CAD build for the part. Positions are in the model's coordinates, mm. Coordinates: 2 decimals unless noted, no trailing zeros. Write each loop counter-clockwise with the first axis right and the second up, starting at its lowest first coordinate (ties: lowest second). Pieces come first, ordered by that corner, then holes. Notation, with made-up numbers: (81, -8) -> (132, -8) arc R24 cw to (132, 23) -> close; hole circle Ø8 at (-28, 69). An arc over 180 degrees is marked (long way). Answer as CSV lines item,"result".
Autodesk Inventor part; units mm, degrees
ref_plane "YZ Plane" through (0, 0, 0) normal (1, 0, 0) x (0, 1, 0)
ref_plane "XZ Plane" through (0, 0, 0) normal (0, 1, 0) x (-1, 0, 0)
ref_plane "XY Plane" through (0, 0, 0) normal (0, 0, 1) x (1, 0, 0)
sketch "Sketch1" plane through (0, 0, 0) normal (1, 0, 0) x (0, 1, 0)
  line L0 (21.2, 0) -> (21.2, -3)
  line L1 (42.4, 0) -> (42.4, -3)
  line L2 (63.6, 0) -> (63.6, -3)
  line L3 (84.8, 0) -> (84.8, -3)
  line L4 (-3, -21.2) -> (3, -21.2)
  line L5 (-3, -42.4) -> (3, -42.4)
  line L6 (-3, -63.6) -> (3, -63.6)
  line L7 (-3, -84.8) -> (3, -84.8)
  line L8 (21.2, -106) -> (21.2, -103)
  line L9 (42.4, -106) -> (42.4, -103)
  line L10 (63.6, -106) -> (63.6, -103)
  line L11 (84.8, -106) -> (84.8, -103)
  line L12 (109, -84.8) -> (103, -84.8)
  line L13 (109, -63.6) -> (103, -63.6)
  line L14 (109, -42.4) -> (103, -42.4)
  line L15 (109, -21.2) -> (103, -21.2)
  line L16 (3, -103) -> (3, -84.8)
  line L17 (3, -63.6) -> (3, -42.4)
  line L18 (3, -21.2) -> (3, -3)
  line L19 (103, -3) -> (103, -21.2)
  line L20 (103, -42.4) -> (103, -63.6)
  line L21 (103, -84.8) -> (103, -103)
  line L22 (21.2, -103) -> (3, -103)
  line L23 (84.8, -106) -> (63.6, -106)
  line L24 (42.4, -106) -> (21.2, -106)
  line L25 (103, -103) -> (84.8, -103)
  line L26 (63.6, -103) -> (42.4, -103)
  line L27 (103, -3) -> (103, 0)
  line L28 (3, -3) -> (3, 0)
  line L29 (3, 0) -> (21.2, 0)
  line L30 (21.2, -3) -> (42.4, -3)
  line L31 (63.6, -3) -> (84.8, -3)
  line L32 (42.4, 0) -> (63.6, 0)
  line L33 (84.8, 0) -> (103, 0)
  line L34 (-3, -21.2) -> (-3, -42.4)
  line L35 (-3, -63.6) -> (-3, -84.8)
  line L36 (109, -84.8) -> (109, -63.6)
  line L37 (109, -42.4) -> (109, -21.2)
  line L38 (0, -26.8) -> (-1, -26.8)
  line L39 (-1, -26.8) -> (-1, -36.8)
  line L40 (-1, -36.8) -> (0, -36.8)
  line L41 (0, -36.8) -> (0, -26.8)
  line L42 (107, -26.8) -> (106, -26.8)
  line L43 (106, -26.8) -> (106, -36.8)
  line L44 (106, -36.8) -> (107, -36.8)
  line L45 (107, -36.8) -> (107, -26.8)
  line L46 (-1, -69.2) -> (0, -69.2)
  line L47 (0, -69.2) -> (0, -79.2)
  line L48 (0, -79.2) -> (-1, -79.2)
  line L49 (-1, -79.2) -> (-1, -69.2)
  line L50 (106, -69.2) -> (105, -69.2)
  line L51 (105, -69.2) -> (105, -79.2)
  line L52 (105, -79.2) -> (106, -79.2)
  line L53 (106, -79.2) -> (106, -69.2)
  point P0 (0, 0)
  dimension "d94" = 1
  dimension "d95" = 10
  dimension "d96" = 1
  dimension "d97" = 10
  dimension "d98" = 10
  dimension "d99" = 1
  dimension "d100" = 10
extrude "Extrusion1" add sketch "Sketch1" along normal blind 3
sketch "Sketch3" plane through (3, 0, 0) normal (1, 0, 0) x (0, 0, -1)
  circle A0 centre (25, 20) radius 1.5
  point P0 (0, 0)
  dimension "d22" = 3
hole "Hole2" at (3, 20, -25) direction (-1, 0, 0) diameter 3 end through all
sketch "Sketch4" plane through (3, 0, 0) normal (1, 0, 0) x (0, 0, -1)
  circle A0 centre (25, 53) radius 1.5
  point P0 (0, 0)
  dimension "d30" = 3
hole "Hole3" at (3, 53, -25) direction (-1, 0, 0) diameter 3 end through all
sketch "Sketch5" plane through (3, 0, 0) normal (1, 0, 0) x (0, 0, -1)
  circle A0 centre (25, 86) radius 1.5
  point P0 (0, 0)
  dimension "d38" = 3
hole "Hole4" at (3, 86, -25) direction (-1, 0, 0) diameter 3 end through all
sketch "Sketch6" plane through (3, 0, 0) normal (1, 0, 0) x (0, 0, -1)
  circle A0 centre (53, 20) radius 1.5
  point P0 (0, 0)
  dimension "d46" = 3
hole "Hole5" at (3, 20, -53) direction (-1, 0, 0) diameter 3 end through all
sketch "Sketch7" plane through (3, 0, 0) normal (1, 0, 0) x (0, 0, -1)
  circle A0 centre (53, 53) radius 1.5
  point P0 (0, 0)
  dimension "d54" = 3
hole "Hole6" at (3, 53, -53) direction (-1, 0, 0) diameter 3 end through all
sketch "Sketch8" plane through (3, 0, 0) normal (1, 0, 0) x (0, 0, -1)
  circle A0 centre (53, 86) radius 1.5
  point P0 (0, 0)
  dimension "d62" = 3
hole "Hole7" at (3, 86, -53) direction (-1, 0, 0) diameter 3 end through all
sketch "Sketch9" plane through (3, 0, 0) normal (1, 0, 0) x (0, 0, -1)
  circle A0 centre (81, 20) radius 1.5
  point P0 (0, 0)
  dimension "d70" = 3
hole "Hole8" at (3, 20, -81) direction (-1, 0, 0) diameter 3 end through all
sketch "Sketch10" plane through (3, 0, 0) normal (1, 0, 0) x (0, 0, -1)
  circle A0 centre (81, 53) radius 1.5
  point P0 (0, 0)
  dimension "d78" = 3
hole "Hole9" at (3, 53, -81) direction (-1, 0, 0) diameter 3 end through all
sketch "Sketch11" plane through (3, 0, 0) normal (1, 0, 0) x (0, 0, -1)
  circle A0 centre (81, 86) radius 1.5
  point P0 (0, 0)
  dimension "d86" = 3
hole "Hole10" at (3, 86, -81) direction (-1, 0, 0) diameter 3 end through all
properties part number "Box side 3" material "PMMA Plastic"
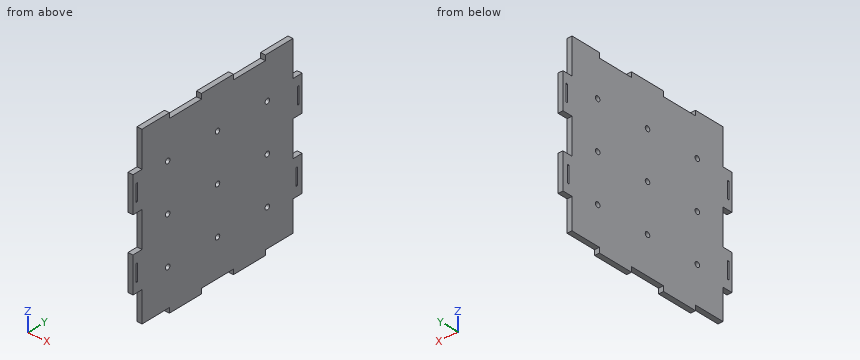
Item 1: Wall check: line 1 (Y direction, x = 1.7, z = -25); line 2 (Z direction, x = 1.9, y = 20); line 3 (Y direction, x = 1.7, z = -53). Give the ranges that are in metal, low to high. Write a range as from..to.
Answer below:
line 1,"y = -3..18.5, 21.5..51.5, 54.5..84.5, 87.5..109"
line 2,"z = -103..-82.5, -79.5..-54.5, -51.5..-26.5, -23.5..0"
line 3,"y = 3..18.5, 21.5..51.5, 54.5..84.5, 87.5..103"
Item 2: Saw through at A-A on y = 53. Give the cut face in (x, z), and give its area (3 significant figures).
Answer below:
outline,"(0, -103) -> (3, -103) -> (3, -82.5) -> (0, -82.5) -> close; (0, -79.5) -> (3, -79.5) -> (3, -54.5) -> (0, -54.5) -> close; (0, -51.5) -> (3, -51.5) -> (3, -26.5) -> (0, -26.5) -> close; (0, -23.5) -> (3, -23.5) -> (3, 0) -> (0, 0) -> close"
area,"282 mm2"
Item 3: Saw through at C-C on x = 2.15. State how many separate pieces and enclosed holes the cut face has, and give its area (3 significant figures).
Answer below:
separate pieces,"1"
enclosed holes,"13"
area,"10,700 mm2"
Item 4: Saw through at B-B on z = -25. Give the cut face in (x, y), and give its area (3 significant figures).
Answer below:
outline,"(0, -3) -> (3, -3) -> (3, 18.5) -> (0, 18.5) -> close; (0, 21.5) -> (3, 21.5) -> (3, 51.5) -> (0, 51.5) -> close; (0, 54.5) -> (3, 54.5) -> (3, 84.5) -> (0, 84.5) -> close; (0, 87.5) -> (3, 87.5) -> (3, 109) -> (0, 109) -> close"
area,"309 mm2"
Item 5: Flat gauge pins, fed straight in: pin 1 (1.5 mm diameter, centred on x = 1.5, y = -1.5, fed in from +Z); pin 2 (1.5 mm diameter, centred on x = 2, z = -1.5, fed in from -Y); pin 3 (0.9 mm diameter, centred on x = 1, z = -104.5, fed in from -Y); pin 4 (2.5 mm diameter, centred on y = 53, z = -81, fed in from -X). Where does each tip first touch, or does it go through?
Answer below:
pin 1,"stops at z = -21.2"
pin 2,"stops at y = 3"
pin 3,"stops at y = 21.2"
pin 4,"passes through"
